Check sheet for the modelled part. Datum: model origin and axes. Units: mm. Round coordinates to 2 decimals unless told otherwise and drop trailing zeros. Loops run counter-clockwise (first coordinate to the right, second up) from the corner with the lowest first, then second, coordinate; pieces in that order, holes last. Notation, with made-up numbers: (50, 18) - (85, 18) arc R17 cw to (85, 26) - close; hole circle Ø6 at (62, 41.5). An arc over 180 degrees is marked (long way). Put each result on its own line as item: value.
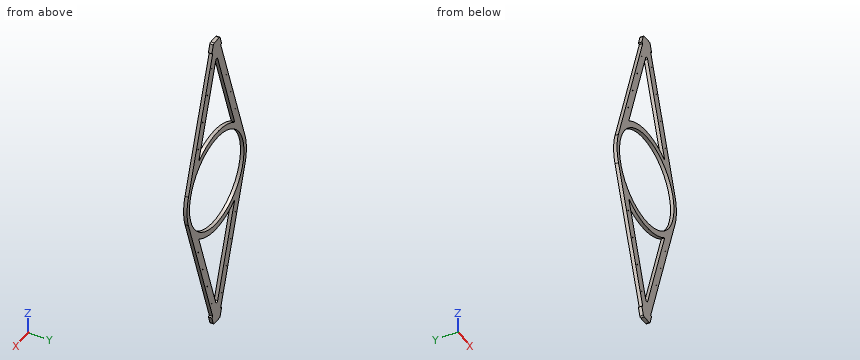
```python
from build123d import *

# Parameters (mm, degrees)
SKETCH2_R           = 2.5
SKETCH2_R_2         = 275
BOSS_EXTRUDE1_DEPTH = 20
CUT_EXTRUDE1_DEPTH  = 21


with BuildPart() as part:
    # Sketch2 → Boss-Extrude1 (new body)
    with BuildSketch(Plane(origin=(0, 0, 0), x_dir=(1, 0, 0), z_dir=(0, 1, 0))):
        with BuildLine():
            Line((-34.517430478, 903.068960265), (-295.040344804, 95.1377682))
            ThreePointArc((-295.040344804, 95.1377682), (-310, 0), (-295.040344804, -95.1377682))
            Line((-295.040344804, -95.1377682), (-34.517430478, -903.068960265))
            ThreePointArc((-34.517430478, -903.068960265), (-30.886866626, -908.083613135), (-25, -910))
            Line((-25, -910), (25, -910))
            ThreePointArc((25, -910), (30.886866626, -908.083613135), (34.517430478, -903.068960265))
            Line((34.517430478, -903.068960265), (295.040344804, -95.1377682))
            ThreePointArc((295.040344804, -95.1377682), (310, 0), (295.040344804, 95.1377682))
            Line((295.040344804, 95.1377682), (34.517430478, 903.068960265))
            ThreePointArc((34.517430478, 903.068960265), (30.886866626, 908.083613135), (25, 910))
            Line((25, 910), (-25, 910))
            ThreePointArc((-25, 910), (-30.886866626, 908.083613135), (-34.517430478, 903.068960265))
        make_face()
        with Locations((-48.373467006, -762.345774842)):
            Circle(SKETCH2_R, mode=Mode.SUBTRACT)
        with Locations((-94.407870974, -619.584317679)):
            Circle(SKETCH2_R, mode=Mode.SUBTRACT)
        with Locations((-140.442274942, -476.822860516)):
            Circle(SKETCH2_R, mode=Mode.SUBTRACT)
        with BuildLine():
            ThreePointArc((-181.680791071, -251.181388952), (0, -310), (181.680791071, -251.181388952))
            Line((181.680791071, -251.181388952), (9.517430478, -785.092770658))
            ThreePointArc((9.517430478, -785.092770658), (0, -792.023810393), (-9.517430478, -785.092770658))
            Line((-9.517430478, -785.092770658), (-181.680791071, -251.181388952))
        make_face(mode=Mode.SUBTRACT)
        with Locations((-186.476678909, -334.061403353)):
            Circle(SKETCH2_R, mode=Mode.SUBTRACT)
        with Locations((48.373467006, -762.345774842)):
            Circle(SKETCH2_R, mode=Mode.SUBTRACT)
        with Locations((94.407870974, -619.584317679)):
            Circle(SKETCH2_R, mode=Mode.SUBTRACT)
        with Locations((140.442274942, -476.822860516)):
            Circle(SKETCH2_R, mode=Mode.SUBTRACT)
        with Locations((186.476678909, -334.061403353)):
            Circle(SKETCH2_R, mode=Mode.SUBTRACT)
        with Locations((-186.476678909, 334.061403353)):
            Circle(SKETCH2_R, mode=Mode.SUBTRACT)
        with Locations((-140.442274942, 476.822860516)):
            Circle(SKETCH2_R, mode=Mode.SUBTRACT)
        with Locations((-94.407870974, 619.584317679)):
            Circle(SKETCH2_R, mode=Mode.SUBTRACT)
        with BuildLine():
            ThreePointArc((181.680791071, 251.181388952), (0, 310), (-181.680791071, 251.181388952))
            Line((-181.680791071, 251.181388952), (-9.517430478, 785.092770658))
            ThreePointArc((-9.517430478, 785.092770658), (0, 792.023810393), (9.517430478, 785.092770658))
            Line((9.517430478, 785.092770658), (181.680791071, 251.181388952))
        make_face(mode=Mode.SUBTRACT)
        with Locations((-48.373467006, 762.345774842)):
            Circle(SKETCH2_R, mode=Mode.SUBTRACT)
        Circle(SKETCH2_R_2, mode=Mode.SUBTRACT)
        with Locations((186.476678909, 334.061403353)):
            Circle(SKETCH2_R, mode=Mode.SUBTRACT)
        with Locations((140.442274942, 476.822860516)):
            Circle(SKETCH2_R, mode=Mode.SUBTRACT)
        with Locations((94.407870974, 619.584317679)):
            Circle(SKETCH2_R, mode=Mode.SUBTRACT)
        with Locations((48.373467006, 762.345774842)):
            Circle(SKETCH2_R, mode=Mode.SUBTRACT)
    extrude(amount=BOSS_EXTRUDE1_DEPTH)

    # Sketch3 → Cut-Extrude1 (cut, through all)
    with BuildSketch(Plane(origin=(0, 20, 0), x_dir=(1, 0, 0), z_dir=(0, 1, 0))):
        with BuildLine():
            Line((-295.040344804, -95.1377682), (-49.523523643, -856.532206403))
            Line((-49.523523643, -856.532206403), (-40.006093165, -853.463246139))
            Line((-40.006093165, -853.463246139), (-285.522914326, -92.068807935))
            ThreePointArc((-285.522914326, -92.068807935), (-300, 0), (-285.522914326, 92.068807935))
            Line((-285.522914326, 92.068807935), (-40.006093165, 853.463246139))
            Line((-40.006093165, 853.463246139), (-49.523523643, 856.532206403))
            Line((-49.523523643, 856.532206403), (-295.040344804, 95.1377682))
            ThreePointArc((-295.040344804, 95.1377682), (-310, 0), (-295.040344804, -95.1377682))
        make_face()
        with BuildLine():
            Line((295.040344804, 95.1377682), (49.523523643, 856.532206403))
            Line((49.523523643, 856.532206403), (40.006093165, 853.463246139))
            Line((40.006093165, 853.463246139), (285.522914326, 92.068807935))
            ThreePointArc((285.522914326, 92.068807935), (300, 0), (285.522914326, -92.068807935))
            Line((285.522914326, -92.068807935), (40.006093165, -853.463246139))
            Line((40.006093165, -853.463246139), (49.523523643, -856.532206403))
            Line((49.523523643, -856.532206403), (295.040344804, -95.1377682))
            ThreePointArc((295.040344804, -95.1377682), (310, 0), (295.040344804, 95.1377682))
        make_face()
    extrude(amount=-CUT_EXTRUDE1_DEPTH, mode=Mode.SUBTRACT)


solid = part.part
```
Item 1: Thickness scan on line 1 (X direction, y = 7.5, z = 316); line 2 (X direction, y = 6.5, z = 537); line 3 (X direction, y = 3.5, z = 818). Record the ranges inside material, lowest first. Write a range as from..to.
Filled sheet:
line 1: -213.31..-160.78, 160.78..213.31
line 2: -142.05..-89.52, 89.52..142.05
line 3: -51.44..51.44
Item 2: Go/stop test with flat-tipped pins: pin 1 (4.5 mm diameter, centred on x = -186.48, z = -334.06, fed in from +Y); pin 2 (8 mm diameter, centred on y = 10.5, z = 491, fed in from +X); pin 3 (12 mm diameter, centred on y = 8, z = -190, fed in from -X). Record where each tip stops, or that it passes through.
Filled sheet:
pin 1: through
pin 2: x = 158.17
pin 3: x = -255.88
Item 3: Section check C-C on y = 10.5. Count the separate pieces of the cut face and the enclosed holes in it, then the cut area to 3 significant figures.
Filled sheet:
separate pieces: 1
enclosed holes: 19
area: 201,000 mm²
Item 4: Section check B-B on z = -701.5. Enter the section's corners in (x, y), then the cut area to 3 significant figures.
Filled sheet:
outline: (-89.01, 0) - (-36.47, 0) - (-36.47, 20) - (-89.01, 20) - close; (36.47, 0) - (89.01, 0) - (89.01, 20) - (36.47, 20) - close
area: 2,100 mm²
Item 5: Section check A-A on z = 0. Enter the section's corners in (x, y).
Filled sheet:
outline: (-300, 0) - (-275, 0) - (-275, 20) - (-300, 20) - close; (275, 0) - (300, 0) - (300, 20) - (275, 20) - close
